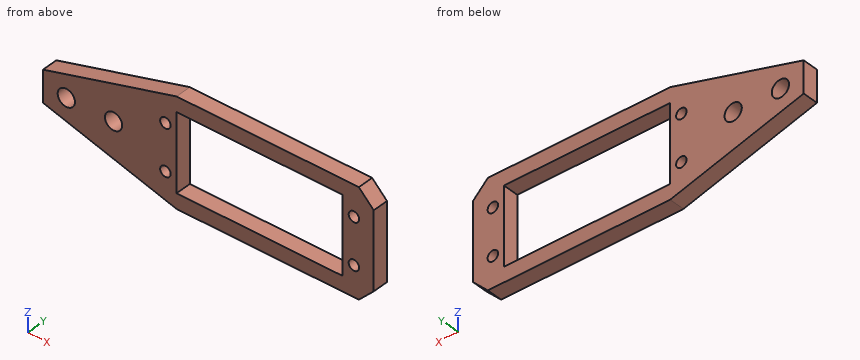
```python
from build123d import *

# Parameters (mm, degrees)
SKETCH1_R           = 2.1082
SKETCH1_R_2         = 3.475
SKETCH1_W           = 67
SKETCH1_H           = 31
BOSS_EXTRUDE1_DEPTH = 6.35


with BuildPart() as part:
    # Sketch1 → Boss-Extrude1 (new body)
    with BuildSketch(Plane(origin=(0, 0, 0), x_dir=(1, 0, 0), z_dir=(0, 1, 0))):
        Polygon((60.675, -21.5), (-12.825, -21.5), (-66.675, -6.35), (-66.675, 6.35), (-12.825, 21.5), (60.675, 21.5), (66.675, 15.5), (66.675, -15.5), align=None)
        with Locations(Location((58.675, 9.25, 0), (0, 0, 270))):
            Circle(SKETCH1_R, mode=Mode.SUBTRACT)
        with Locations(Location((58.675, -9.25, 0), (0, 0, 90))):
            Circle(SKETCH1_R, mode=Mode.SUBTRACT)
        with Locations(Location((-17.325, -9.25, 0), (0, 0, 270))):
            Circle(SKETCH1_R, mode=Mode.SUBTRACT)
        with Locations(Location((-17.325, 9.25, 0), (0, 0, 90))):
            Circle(SKETCH1_R, mode=Mode.SUBTRACT)
        with Locations(Location((-57.275, 0, 0), (0, 0, 270))):
            Circle(SKETCH1_R_2, mode=Mode.SUBTRACT)
        with Locations(Location((-38.225, 0, 0), (0, 0, 270))):
            Circle(SKETCH1_R_2, mode=Mode.SUBTRACT)
        with Locations((20.675, 0)):
            Rectangle(SKETCH1_W, SKETCH1_H, mode=Mode.SUBTRACT)
    extrude(amount=BOSS_EXTRUDE1_DEPTH)


solid = part.part
```
Work out the finished part from the listing and answer in its coordinate system (mm). Give positions to 0.01 mm unless a question says otherwise; leave off trailing zeros. Loops run counter-clockwise (first coordinate to the right, second up) from the corner with the lowest first, then second, coordinate; pieces in that order, holes last. Notation, with made-up numbers: (87, -8.75) -> (122, -8.75) arc R25 cw to (122, 16.25) -> close; hole circle Ø5 at (0, 49). An arc over 180 degrees is marked (long way). Write item = value, one per line. Start each with the question number.
(1) Find section B-B on z = 0. Give the vertices of the cut face in (x, y) (3 decimals).
(2) Find section C-C on y = 1.5. Give the vertices of the cut face in (x, z) (3 decimals), and give its area (3 significant figures).
(3) Find section A-A on x = 26. Give the vertices of the cut face in (y, z), and give its area (3 significant figures).
(4) Given pin 1 Ø3 at (x, y) = (-15.5, 3.5) entering from +Z, flat-ended and moving along its own axis, determine where the tip first touches the part or whether it passes through.
(5) Find the intervals of material crossed by probe 1 along X at (y, z) = (4.75, 0) (3 decimals); probe 2 along X at (y, z) = (0.5, 5) (3 decimals); probe 3 along Z at (x, y) = (5, 5.75), in increasing order. Write a range as from..to.
(6) Find section D-D on z = 9.25. Give the vertices of the cut face in (x, y) (3 decimals).
From the geometry:
q1.outline = (-66.675, 0) -> (-60.75, 0) -> (-60.75, 6.35) -> (-66.675, 6.35) -> close; (-53.8, 0) -> (-41.7, 0) -> (-41.7, 6.35) -> (-53.8, 6.35) -> close; (-34.75, 0) -> (-12.825, 0) -> (-12.825, 6.35) -> (-34.75, 6.35) -> close; (54.175, 0) -> (66.675, 0) -> (66.675, 6.35) -> (54.175, 6.35) -> close
q2.outline = (-66.675, -6.35) -> (-12.825, -21.5) -> (60.675, -21.5) -> (66.675, -15.5) -> (66.675, 15.5) -> (60.675, 21.5) -> (-12.825, 21.5) -> (-66.675, 6.35) -> close; hole circle Ø6.95 at (-57.275, 0); hole circle Ø6.95 at (-38.225, 0); hole circle Ø4.216 at (-17.325, -9.25); hole circle Ø4.216 at (-17.325, 9.25); hole (-12.825, -15.5) -> (54.175, -15.5) -> (54.175, 15.5) -> (-12.825, 15.5) -> close; hole circle Ø4.216 at (58.675, -9.25); hole circle Ø4.216 at (58.675, 9.25)
q2.area = 2,670 mm^2
q3.outline = (0, -21.5) -> (6.35, -21.5) -> (6.35, -15.5) -> (0, -15.5) -> close; (0, 15.5) -> (6.35, 15.5) -> (6.35, 21.5) -> (0, 21.5) -> close
q3.area = 76.2 mm^2
q4.pin_1 = 21.17
q5.probe_1 = -66.675..-60.75, -53.8..-41.7, -34.75..-12.825, 54.175..66.675
q5.probe_2 = -66.675..-12.825, 54.175..66.675
q5.probe_3 = -21.5..-15.5, 15.5..21.5
q6.outline = (-56.367, 0) -> (-19.433, 0) -> (-19.433, 6.35) -> (-56.367, 6.35) -> close; (-15.217, 0) -> (-12.825, 0) -> (-12.825, 6.35) -> (-15.217, 6.35) -> close; (54.175, 0) -> (56.567, 0) -> (56.567, 6.35) -> (54.175, 6.35) -> close; (60.783, 0) -> (66.675, 0) -> (66.675, 6.35) -> (60.783, 6.35) -> close
